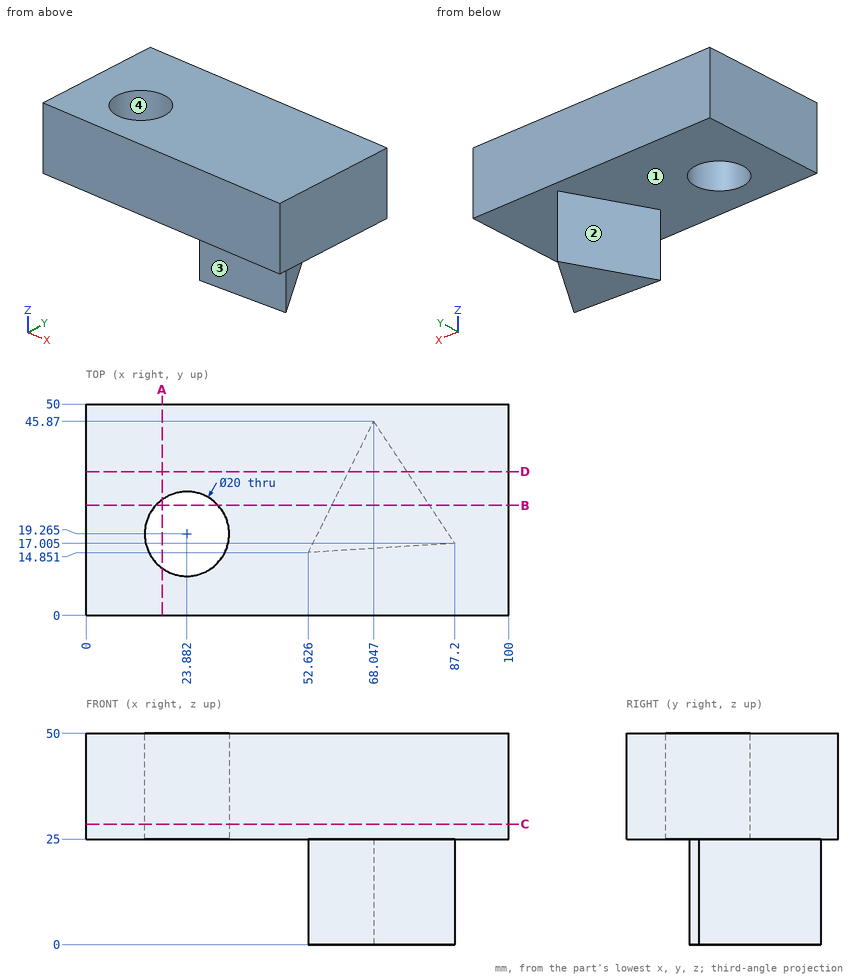
Input: dimensioned drawing with shaded views. Units: mm. Origin: part minimum x, y, z. Give positions to 0.01 mm unless a question says otherwise; leave off trailing zeros. Write each loop counter-clockwise with the first axis right and the second up, starting at its lowest first coordinate (ties: lowest second). Pieces come first, ordered by that corner, then holes.
Q1. Section C-C, the plane z = 28.5. Output: boundary loops of the cut face in (x, y) (1 decimal), plus the area to 3 significant figures.
Q2. Section A-A, the plane x = 18. Output: boundary loops of the cut face in (y, z), plus the area to 3 significant figures.
Q3. Section D-D, the plane y = 34. Output: boundary loops of the cut face in (x, z).
Q4. First-contact query: P1, Ø15, axis at x = 32, y = 29, coming from the -Z side; P2, Ø6, axis at y = 41, z = 6, coming from the +X side; P3, Ø4, axis at y = 27.5, z = 14, coming from the -X side; P4, Ø16, axis at x = 23.88, y = 19.26, coming from the -Z side. Flat tips, straight axial feed; report the tip coordinate or a pass-through.
Q5. Material intervals for probe 1 along Z at (x, y) = (79.5, 12); probe 2 along X at (y, z) = (17, 26); probe 3 along Y at (x, z) = (58, 15.5) (1 decimal), sorted ascending.
Q6. Pull-direction query (X, two-part tool) for the marked faces 1, 2, 3 and 4; classes: pulls with the +X half, pulls with the -X half, needs draft (parallel to the pull), parting line crosses it, or undercut.
Q7. Section B-B, the plane y = 26. Output: boundary loops of the cut face in (x, z), plus the area to 3 significant figures.
Filled in:
1. outline: (0, 0) - (100, 0) - (100, 50) - (0, 50) - close; hole circle Ø20 at (23.9, 19.3)
1. area: 4,690 mm2
2. outline: (0, 25) - (11.18, 25) - (11.18, 50) - (0, 50) - close; (27.35, 25) - (50, 25) - (50, 50) - (27.35, 50) - close
2. area: 846 mm2
3. outline: (0, 25) - (62.15, 25) - (62.15, 0) - (75.92, 0) - (75.92, 25) - (100, 25) - (100, 50) - (0, 50) - close
4. P1: stops at z = 25
4. P2: stops at x = 73.27
4. P3: stops at x = 57.92
4. P4: passes through
5. probe 1: z = 25 to 50
5. probe 2: x = 0 to 14.14, 33.62 to 100
5. probe 3: y = 15.2 to 25.7
6. face 1: needs draft
6. face 2: pulls with the -X half
6. face 3: pulls with the +X half
6. face 4: undercut
7. outline: (0, 25) - (16.49, 25) - (16.49, 50) - (0, 50) - close; (31.27, 25) - (58.17, 25) - (58.17, 0) - (81.23, 0) - (81.23, 25) - (100, 25) - (100, 50) - (31.27, 50) - close
7. area: 2,710 mm2
